Autodesk Inventor part; units mm, degrees
ref_plane "YZ Plane" through (0, 0, 0) normal (1, 0, 0) x (0, 1, 0)
ref_plane "XZ Plane" through (0, 0, 0) normal (0, 1, 0) x (-1, 0, 0)
ref_plane "XY Plane" through (0, 0, 0) normal (0, 0, 1) x (1, 0, 0)
sketch "Эскиз1" plane through (0, 0, 0) normal (0, 1, 0) x (-1, 0, 0)
  line L0 (17.4798, -42.1371) -> (-42.5202, -42.1371)
  line L1 (-42.5202, -42.1371) -> (-42.5202, -82.1371)
  line L2 (-42.5202, -82.1371) -> (-22.5202, -82.1371)
  line L3 (-22.5202, -82.1371) -> (-22.5202, -62.1371)
  line L4 (-22.5202, -62.1371) -> (-2.5202, -62.1371)
  line L5 (-2.5202, -62.1371) -> (-2.5202, -82.1371)
  line L6 (-2.5202, -82.1371) -> (17.4798, -82.1371)
  line L7 (17.4798, -82.1371) -> (17.4798, -42.1371)
  point P0 (0, 0)
  dimension "d1" = 40
  dimension "d3" = 20
  dimension "d4" = 20
  dimension "d5" = 20
extrude "Выдавливание1" add sketch "Эскиз1" along normal blind 20
fillet "Сопряжение1" radius 2 14 edges at (-17.4798, 20, -62.1371) (12.5202, 20, -42.1371) (2.5202, 20, -72.1371) (12.5202, 20, -62.1371) (-7.4798, 20, -82.1371) (22.5202, 20, -72.1371) (32.5202, 20, -82.1371) (42.5202, 20, -62.1371) (42.5202, 10, -82.1371) (2.5202, 10, -82.1371) (22.5202, 10, -82.1371) (-17.4798, 10, -82.1371) (-17.4798, 10, -42.1371) (42.5202, 10, -42.1371)
sketch "Эскиз2" plane through (0, 0, 0) normal (0, -1, 0) x (1, 0, 0)
  line L0 (-15.4798, -42.1371) -> (40.5202, -42.1371)
  point P0 (0, 0)
  point P1 (32.9606, -52.1371)
  point P2 (-7.0394, -52.1371)
  dimension "d9" = 40
  dimension "d10" = 10
hole "Отверстие1" at (32.9606, 0, -52.1371) at (-7.0394, 0, -52.1371) direction (0, 1, 0) diameter 3 depth 10 tip angle 90
properties part number "stand_stop"
Model file for the job. Use its own axes, mm. A direction names the side the tool comes from. Give positions to 0.01 mm unless a question says otherwise; leave off trailing zeros. Loops run counter-clockwise (first coordinate to the right, second up) from the corner with the lowest first, then second, coordinate; pieces in that order, holes last. Notation, with made-up numbers: (1.25, 10) - (52.25, 10) arc R26 ccw to (52.25, 44) - close; hole circle Ø9 at (-36, -38). An arc over 180 degrees is marked (long way). One line per item, written item: value. Start each with the question number.
1. Slice it at A-A (z = -70.5). List the corners of the cut face in (x, y).
2. Which spindle directions (+Z, -Z, +X, -X, +Y, -Y) get a long thin tool onto all of the face, cutting with end or side? Do faces 1 (the cylindrical face through (33.873, 5.07, -50.947)), 2 (the flat face through (13, 9, -62.137)), 3 (the cylindrical face through (41.95, 9.126, -81.536)). Say none if no direction does.
3. Pull direction Z, two halves, no side cores. Call faces 4 (the flat face through (-7, 9, -82.137)), 5 (the cylindrical face through (-6.127, 5.07, -50.947)), 6 (the cylindrical face through (-16.91, 9.13, -42.74)), 7 (the flat face through (12.9, 0, -61.9)): pulls with the +Z half, pulls with the -Z half, needs draft (parallel to the pull), parting line crosses it, or undercut.
4. Slice it at D-D (x = 7). List the corners of the cut face in (y, z), plus the area to 3 significant figures.
5. Slice it at C-C (y = 13). List the corners of the cut face in (x, z).
6. Pin check, flat tip, straight feed: pin 1 (5.5 mm diameter, centred on x = 14.5, y = 11.5, fed in from -Z). Stop position of the tip, or through.
7. Slice it at B-B (y = 3.75). List the corners of the cut face in (x, z), plus the area to 3 significant figures.
8. Probe L1, parallel to X at y = 5.75, z = -65; L2, parallel to X at y = 9, z = -51.5; L3, parallel to X at y = 5, z = -52.5. List the from-to ranges inside material, lowest first. Write a range as from..to.
Solution:
1. outline: (-17.48, 0) - (2.52, 0) - (2.52, 18) arc R2 ccw to (0.52, 20) - (-15.48, 20) arc R2 ccw to (-17.48, 18) - close; (22.52, 0) - (42.52, 0) - (42.52, 18) arc R2 ccw to (40.52, 20) - (24.52, 20) arc R2 ccw to (22.52, 18) - close
2. face 1: -Y
2. face 2: -Z, +Y, -Y
2. face 3: -Z, +X, +Y, -Y
3. face 4: pulls with the -Z half
3. face 5: undercut
3. face 6: pulls with the +Z half
3. face 7: needs draft
4. outline: (0, -62.14) - (18, -62.14) arc R2 ccw to (20, -60.14) - (20, -44.14) arc R2 ccw to (18, -42.14) - (0, -42.14) - close
4. area: 398 mm^2
5. outline: (-17.48, -80.14) arc R2 ccw to (-15.48, -82.14) - (0.52, -82.14) arc R2 ccw to (2.52, -80.14) - (2.52, -62.14) - (22.52, -62.14) - (22.52, -80.14) arc R2 ccw to (24.52, -82.14) - (40.52, -82.14) arc R2 ccw to (42.52, -80.14) - (42.52, -44.14) arc R2 ccw to (40.52, -42.14) - (-15.48, -42.14) arc R2 ccw to (-17.48, -44.14) - close
6. pin 1: stops at z = -62.14
7. outline: (-17.48, -80.14) arc R2 ccw to (-15.48, -82.14) - (0.52, -82.14) arc R2 ccw to (2.52, -80.14) - (2.52, -62.14) - (22.52, -62.14) - (22.52, -80.14) arc R2 ccw to (24.52, -82.14) - (40.52, -82.14) arc R2 ccw to (42.52, -80.14) - (42.52, -44.14) arc R2 ccw to (40.52, -42.14) - (-15.48, -42.14) arc R2 ccw to (-17.48, -44.14) - close; hole circle Ø3 at (-7.04, -52.14); hole circle Ø3 at (32.96, -52.14)
7. area: 1,980 mm^2
8. L1: x = -17.48..2.52, 22.52..42.52
8. L2: x = -17.48..-8.4, -5.68..31.6, 34.32..42.52
8. L3: x = -17.48..-8.49, -5.58..31.51, 34.42..42.52
